Autodesk Inventor part; units mm, degrees
ref_plane "YZ Plane" through (0, 0, 0) normal (1, 0, 0) x (0, 1, 0)
ref_plane "XZ Plane" through (0, 0, 0) normal (0, 1, 0) x (-1, 0, 0)
ref_plane "XY Plane" through (0, 0, 0) normal (0, 0, 1) x (1, 0, 0)
sketch "Boceto1" plane through (0, 0, 0) normal (0, 1, 0) x (-1, 0, 0)
  circle A0 centre (0, 0) radius 25
  circle A1 centre (0, -20) radius 3
  circle A2 centre (-14.1421, -14.1421) radius 3
  circle A3 centre (14.1421, -14.1421) radius 3
  circle A4 centre (0, 20) radius 3
  circle A5 centre (-14.1421, 14.1421) radius 3
  circle A6 centre (14.1421, 14.1421) radius 3
  line L0 (0, -23) -> (0, -28.5119)
  dimension "d2" = 6
  dimension "d0" = 50
  dimension "d4" = 6
  dimension "d6" = 6
extrude "Extrusión1" add sketch "Boceto1" along normal blind 10
sketch "Boceto2" plane through (0, 10, 0) normal (0, 1, 0) x (1, 0, 0)
  circle A0 centre (0, 0) radius 9.15
  circle A1 centre (0, 0) radius 13
  dimension "d9" = 18.3
  dimension "d10" = 26
extrude "Extrusión2" add sketch "Boceto2" along normal blind 106
fillet "Empalme1" radius 2 1 edges at (-13, 10, 0)
chamfer "Chaflán1" distance 1 angle 45 1 edges at (-9.15, 116, 0)
sketch "Boceto4" plane through (0, 116, 0) normal (0, 1, 0) x (1, 0, 0)
  circle A0 centre (0, 0) radius 11
  circle A1 centre (0, 0) radius 14
  dimension "d22" = 28
extrude "Extrusión4" add sketch "Boceto4" against normal blind 3
fillet "Empalme3" radius 12 1 edges at (-13, 113, 0)
thread "Thread1"
thread "Thread2"
thread "Thread3"
thread "Thread4"
thread "Thread5"
thread "Thread6"
chamfer "Chamfer2" [suppressed]
ref_plane "Work Plane1" through (0, 96, 0) normal (0, 1, 0) x (1, 0, 0)
sketch "Sketch5" plane through (0, 96, 0) normal (0, 1, 0) x (1, 0, 0)
  circle A0 centre (0, 0) radius 13
  circle A1 centre (0, 0) radius 13
  circle A2 centre (0, 0) radius 9.15
  circle A3 centre (0, 0) radius 9.15
  circle A4 centre (0, 0) radius 9.15
  circle A5 centre (0, 0) radius 9.15
  circle A6 centre (0, 0) radius 10.85
  dimension "d43" = 1.7
extrude "Extrusion5" cut sketch "Sketch5" along normal blind 1 contours A6
thread "Thread7"
properties part number "herramienta2"
Geometry: final body of the model. Coordinates: model frame, mm. A direction names the side the tool comes from. Give positions to 0.01 mm unless a question says otherwise; leave off trailing zeros. Loops run counter-clockwise (first coordinate to the right, second up) from the corner with the lowest first, then second, coordinate; pieces in that order, holes last. Notation, with made-up numbers: (33.5, 70) -> (43.5, 70) arc R19 cw to (43.5, 74) -> close; hole circle Ø10 at (78.25, -5.75). An arc over 180 degrees is marked (long way). Use one line per item in the form item = value.
Item 1: Section query C-C on x = 0. Give the number of separate pieces and of enclosed holes in the cut face, and give its area (3 significant figures).
A:
separate_pieces = 3
enclosed_holes = 0
area = 1,200 mm^2
Item 2: Draft query along Y for faces 4 (the face through (-8, 96.49, 7.33)), 5 (the face through (4.919, 52.398, 7.715)), 6 (the face through (-11, 10, -11)). Return one class per face: pulls with the +Y half, pulls with the -Y half, needs draft (parallel to the pull), parting line crosses it, or undercut.
A:
face_4 = undercut
face_5 = needs draft
face_6 = pulls with the +Y half
Item 3: Line query: probe 1 along Z at (x, y) = (0, 4); probe 2 along Y at (x, z) = (4, -10); probe 3 along Z at (x, y) = (-13, 6.5). Output: solid intervals per line, ascending.
A:
probe_1 = -25 to -23, -17 to 17, 23 to 25
probe_2 = 0 to 96, 97 to 116
probe_3 = -21.35 to -16.92, -11.37 to 11.37, 16.92 to 21.35
Item 4: Access query for faces 1 (the face through (-5, 96, 8)), 2 (the face through (0.65, 4.93, 22.93)), 3 (the face through (4.919, 105.874, 7.715)). Directions: +Z, -Z, +X, -X, +Y, -Y. A direction counts if a zero-diameter tool reaches every point of the face in a straight line with its end or side. Return the directions, or none.
A:
face_1 = none
face_2 = +Y, -Y
face_3 = +Y
Item 5: Section query A-A on z = 20. Output: boundary loops of the cut face in (x, y), and give its area (3 significant figures).
A:
outline = (-15, 0) -> (-3, 0) -> (-3, 10) -> (-15, 10) -> close; (3, 0) -> (15, 0) -> (15, 10) -> (3, 10) -> close
area = 240 mm^2
Item 6: Section query D-D on y = 78. Output: boundary loops of the cut face in (x, z), and give its area (3 significant figures).
A:
outline = circle Ø26 at (0, 0); hole circle Ø18.3 at (0, 0)
area = 268 mm^2
Item 7: Section query B-B on z = 0. Output: boundary loops of the cut face in (x, y), and give its area (3 significant figures).
A:
outline = (-25, 0) -> (25, 0) -> (25, 10) -> (15, 10) arc R2 cw to (13, 12) -> (13, 108.2) arc R12 cw to (14, 113) -> (14, 116) -> (10.15, 116) -> (9.15, 115) -> (9.15, 97) -> (10.85, 97) -> (10.85, 96) -> (9.15, 96) -> (9.15, 10) -> (-9.15, 10) -> (-9.15, 96) -> (-10.85, 96) -> (-10.85, 97) -> (-9.15, 97) -> (-9.15, 115) -> (-10.15, 116) -> (-14, 116) -> (-14, 113) arc R12 cw to (-13, 108.2) -> (-13, 12) arc R2 cw to (-15, 10) -> (-25, 10) -> close
area = 1,320 mm^2
Item 8: Pin query (flat end, axial travel): P1, Ø16.5, axis at x = 0, z = 0, coming from the +Y side; P2, Ø4, axis at y = 83.5, z = 7, coming from the -X side; P3, Ø4, axis at y = 90, z = -13, coming from the -X side. Return the tip coordinate at first contact, or that it passes through.
A:
P1 = 10
P2 = -12
P3 = -6.93
